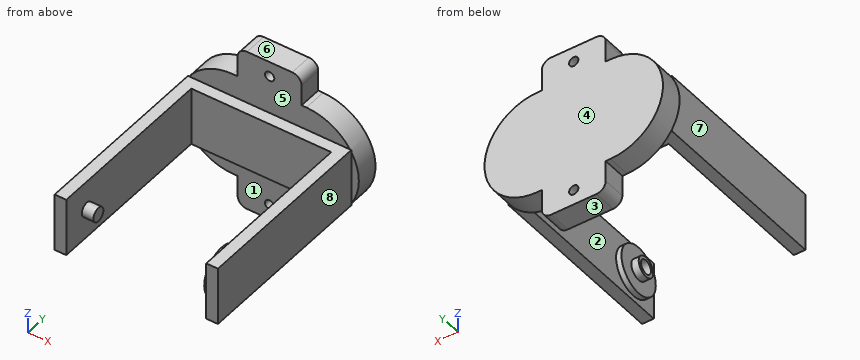
from build123d import *

# Parameters (mm, degrees)
SKETCH_1_W       = 25
SKETCH_1_H       = 80
EXTRUDE_1_DEPTH  = 5
SKETCH_8_W       = 25
SKETCH_8_H       = 5
EXTRUDE_6_DEPTH  = 60
SKETCH_9_W       = 25
SKETCH_9_H       = 80
EXTRUDE_7_DEPTH  = 5
SKETCH_10_R      = 10.3
EXTRUDE_9_DEPTH  = 2.3
SKETCH_12_R      = 4.35
SKETCH_12_R_2    = 3
EXTRUDE_10_DEPTH = 3.15
EXTRUDE_START    = 5
SKETCH_13_R      = 3
EXTRUDE_11_DEPTH = 5
SKETCH_15_R      = 2
EXTRUDE_12_DEPTH = 10


with BuildPart() as part:
    # 草圖1 → 填料-伸長1 (new body)
    with BuildSketch(Plane(origin=(0, 0, 0), x_dir=(0, 0, -1), z_dir=(1, 0, 0))):
        with Locations((0.068306011, -18.756830601)):
            Rectangle(SKETCH_1_W, SKETCH_1_H)
    extrude(amount=EXTRUDE_1_DEPTH)

    # 草圖8 → 填料-伸長6 (add)
    with BuildSketch(Plane(origin=(5, 0, 0), x_dir=(0, 0, -1), z_dir=(1, 0, 0))):
        with Locations((0.068306011, 18.743169399)):
            Rectangle(SKETCH_8_W, SKETCH_8_H)
    extrude(amount=EXTRUDE_6_DEPTH)

    # 草圖9 → 填料-伸長7 (add)
    with BuildSketch(Plane(origin=(65, 0, 0), x_dir=(0, 0, -1), z_dir=(1, 0, 0))):
        with Locations((0.068306011, -18.756830601)):
            Rectangle(SKETCH_9_W, SKETCH_9_H)
    extrude(amount=EXTRUDE_7_DEPTH)

    # 草圖10 → 填料-伸長9 (add)
    with BuildSketch(Plane.ZY.offset(-65)):
        with Locations(Location((-0.068306011, -46.456830601, 0), (0, 0, 180))):
            Circle(SKETCH_10_R)
    extrude(amount=EXTRUDE_9_DEPTH)

    # 草圖12 → 填料-伸長10 (add)
    with BuildSketch(Plane.ZY.offset(-62.7)):
        with Locations((-0.068306011, -46.456830601)):
            Circle(SKETCH_12_R)
        with Locations((-0.068306011, -46.456830601)):
            Circle(SKETCH_12_R_2, mode=Mode.SUBTRACT)
    extrude(amount=EXTRUDE_10_DEPTH)

    # 草圖13 → 填料-伸長11 (add)
    with BuildSketch(Plane(origin=(5, 0, 0), x_dir=(0, 0, -1), z_dir=(1, 0, 0)).offset(EXTRUDE_START)):
        with Locations(Location((0.068306011, -46.456830601, 0), (0, 0, 180))):
            Circle(SKETCH_13_R)
    extrude(amount=-EXTRUDE_11_DEPTH)

    # 草圖15 → 填料-伸長12 (add)
    # profile 1 of 3: a face of its own
    with BuildSketch(Plane(origin=(0, 21.243169399, 0), x_dir=(1, 0, 0), z_dir=(0, 1, 0))):
        with BuildLine():
            Line((19.25, 22.568306011), (50.75, 22.568306011))
            ThreePointArc((50.75, 22.568306011), (73.25, 0.068306011), (50.75, -22.431693989))
            Line((50.75, -22.431693989), (19.25, -22.431693989))
            ThreePointArc((19.25, -22.431693989), (-3.25, 0.068306011), (19.25, 22.568306011))
        make_face()
    # profile 2 of 3: a face of its own
    with BuildSketch(Plane(origin=(0, 21.243169399, 0), x_dir=(1, 0, 0), z_dir=(0, 1, 0))):
        with BuildLine():
            Line((48.7, -22.431693989), (21.3, -22.431693989))
            Line((21.3, -22.431693989), (21.3, -31.431693989))
            ThreePointArc((21.3, -31.431693989), (22.471572875, -34.260121114), (25.3, -35.431693989))
            Line((25.3, -35.431693989), (44.7, -35.431693989))
            ThreePointArc((44.7, -35.431693989), (47.528427125, -34.260121114), (48.7, -31.431693989))
            Line((48.7, -31.431693989), (48.7, -22.431693989))
        make_face()
        with Locations(Location((35, -28.931693989, 0), (0, 0, 270))):
            Circle(SKETCH_15_R, mode=Mode.SUBTRACT)
    # profile 3 of 3: a face of its own
    with BuildSketch(Plane(origin=(0, 21.243169399, 0), x_dir=(1, 0, 0), z_dir=(0, 1, 0))):
        with BuildLine():
            Line((21.3, 22.568306011), (48.7, 22.568306011))
            Line((48.7, 22.568306011), (48.7, 31.568306011))
            ThreePointArc((48.7, 31.568306011), (47.528427125, 34.396733136), (44.7, 35.568306011))
            Line((44.7, 35.568306011), (25.3, 35.568306011))
            ThreePointArc((25.3, 35.568306011), (22.471572875, 34.396733136), (21.3, 31.568306011))
            Line((21.3, 31.568306011), (21.3, 22.568306011))
        make_face()
        with Locations(Location((35, 29.068306011, 0), (0, 0, 270))):
            Circle(SKETCH_15_R, mode=Mode.SUBTRACT)
    extrude(amount=EXTRUDE_12_DEPTH)


solid = part.part
Input: part model. Units: mm. Frame: model coordinates. Face numbers are marked on the shaded views. A direction names the side the tool comes from. Give positions to 0.01 mm unless a question says otherwise; leave off trailing zeros. Write each loop counter-clockwise with the first axis right and the second up, starting at its lowest first coordinate (ties: lowest second). Pieces come first, ordered by that corner, then holes.
Q1. Set-up query: the marked faces 4, 5, 6, 7 and 8. Return all of +Z, -Z, +X, -X, +Y, -Y with unobstructed straight access to the full face (end or side cutting, diameter ignored); none if empty.
Q2. First-contact query: P1, Ø1, axis at x = 13.5, y = 21, coming from the -Z side; P2, Ø1.6, axis at x = 20, y = 25, coming from the +Z side; P3, Ø7.5, axis at y = -7, z = -5.5, coming from the +X side. Flat tips, straight axial feed; report the tip coordinate or a pass-through.
Q3. Section C-C, the plane x = 7.5. Output: boundary loops of the cut face in (y, z).
Q4. Pull-direction query (Y, two-part tool) for the marked faces 1, 2 and 3; classes: pulls with the +Y half, pulls with the -Y half, needs draft (parallel to the pull), parting line crosses it, or undercut.
Q5. Material intervals for probe 1 along X at (y, z) = (-15, -0.5); probe 2 along Y at (x, z) = (53, -11.5); probe 3 along Z at (x, y) = (3.5, -5.5), sorted ascending.
Q6. Section B-B, the plane x = 35. Output: boundary loops of the cut face in (y, z).
Q7. Section D-D, the plane x = 55. Output: boundary loops of the cut face in (y, z).
Q8. Section A-A, the plane y = -8. Output: boundary loops of the cut face in (x, z).
Filled in:
1. face 4: +Z, -Z, +X, -X, +Y
1. face 5: +Z, +X, -X, -Y
1. face 6: +Z, +X, -X, +Y, -Y
1. face 7: +Z, -Z, -X, -Y
1. face 8: +Z, -Z, +X, -Y
2. P1: stops at z = -21.93
2. P2: stops at z = 22.43
2. P3: stops at x = 70
3. outline: circle Ø6 at (-46.46, -0.07); (16.24, -12.57) - (21.24, -12.57) - (21.24, -19.26) - (31.24, -19.26) - (31.24, 19.12) - (21.24, 19.12) - (21.24, 12.43) - (16.24, 12.43) - close
4. face 1: pulls with the -Y half
4. face 2: undercut
4. face 3: needs draft
5. probe 1: x = 0 to 5, 65 to 70
5. probe 2: y = 16.24 to 31.24
5. probe 3: z = -12.57 to 12.43
6. outline: (16.24, -12.57) - (21.24, -12.57) - (21.24, -27.07) - (31.24, -27.07) - (31.24, 26.93) - (21.24, 26.93) - (21.24, 12.43) - (16.24, 12.43) - close; (21.24, -35.57) - (31.24, -35.57) - (31.24, -31.07) - (21.24, -31.07) - close; (21.24, 30.93) - (31.24, 30.93) - (31.24, 35.43) - (21.24, 35.43) - close
7. outline: (16.24, -12.57) - (21.24, -12.57) - (21.24, -22.16) - (31.24, -22.16) - (31.24, 22.03) - (21.24, 22.03) - (21.24, 12.43) - (16.24, 12.43) - close
8. outline: (0, -12.57) - (5, -12.57) - (5, 12.43) - (0, 12.43) - close; (65, -12.57) - (70, -12.57) - (70, 12.43) - (65, 12.43) - close
